Source: CAD feature listing. Evaluate the final solid. Frame: model axes, mm. Face numbers are marked on the shaded views. A direction names the side the tool comes from. Coordinates: 2 decimals unless noted, no trailing zeros. Loops run counter-clockwise (first coordinate to the right, second up) from the corner with the lowest first, then second, coordinate; pieces in that order, holes last.
Item 1: Reachability of the marked faces 1, 2 and 3 from +Z, -Z, +X, -X, +Y, -Y: full face, straight path, thin tool, end or side. Return the list, or none.
Item 2: Pin query (flat end, axial travel): pin 1 Ø8 at (x, y) = (9.5, -2.5) entering from +Z. Return the tip coordinate at first contact, or that it passes through.
Item 3: Line query: probe 1 along X at (y, z) = (-3.25, 11.25) (3 decimals); probe 2 along Y at (x, z) = (3.5, 7.5); probe 3 along Y at (x, z) = (5.5, 9.25). Output: solid intervals per line, ascending.
Item 4: Section query D-D, the plane x = 0. Return the cut outline in (y, z), then the cut area to 3 significant figures.
Item 5: Pull-direction query (Z, two-part tool) for the marked faces 4, 5 and 6; classes: +Z half, -Z half, draft (parallel to the pull), parting line (faces both ways), or undercut.
Item 6: Section query B-B, the plane x = -6.5. Return the cut outline in (y, z), then the cut area to 3 significant figures.
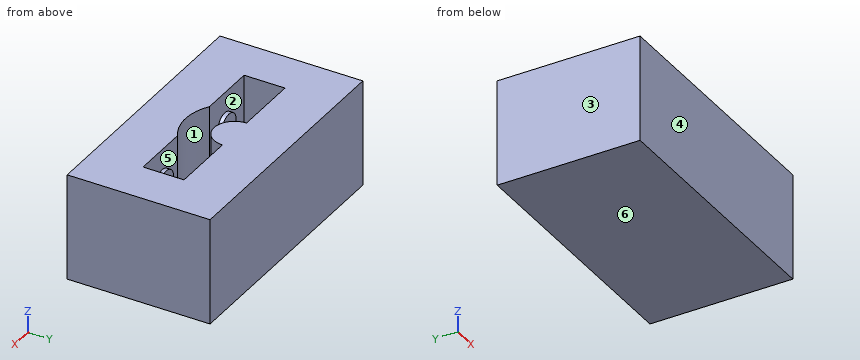
```python
from build123d import *

# Parameters (mm, degrees)
SKETCH1_R      = 24
EXTRUDE1_DEPTH = 5
SKETCH2_R      = 24
EXTRUDE2_DEPTH = 8
SKETCH9_R      = 24
SKETCH9_W      = 31.75
SKETCH9_H      = 17.4625
EXTRUDE4_DEPTH = 13
SKETCH11_R     = 1.5
EXTRUDE6_DEPTH = 0.5


with BuildPart() as part:
    # Sketch1 → Extrude1 (new body)
    with BuildSketch(Plane.XY):
        Circle(SKETCH1_R)
    extrude(amount=EXTRUDE1_DEPTH)

    # Sketch2 → Extrude2 (add)
    with BuildSketch(Plane.XY.offset(5)):
        Circle(SKETCH2_R)
        with BuildLine():
            Line((-2.5, 0), (-10.5, 0))
            Line((-10.5, 0), (-10.5, -5))
            Line((-10.5, -5), (-3.31662479, -5))
            ThreePointArc((-3.31662479, -5), (0, -6), (3.31662479, -5))
            Line((3.31662479, -5), (10.5, -5))
            Line((10.5, -5), (10.5, 0))
            Line((10.5, 0), (2.5, 0))
            ThreePointArc((2.5, 0), (0, -2.5), (-2.5, 0))
        make_face(mode=Mode.SUBTRACT)
    extrude(amount=EXTRUDE2_DEPTH)

    # Sketch9 → Extrude4 (cut)
    with BuildSketch(Plane.XY.offset(13)):
        Circle(SKETCH9_R)
        with Locations((0, -2.38125)):
            Rectangle(SKETCH9_W, SKETCH9_H, mode=Mode.SUBTRACT)
    extrude(amount=-EXTRUDE4_DEPTH, mode=Mode.SUBTRACT)

    # Sketch11 → Extrude6 (add)
    with BuildSketch(Plane(origin=(0, -5, 0), x_dir=(1, 0, 0), z_dir=(0, 1, 0))):
        with Locations((-6.5, -9)):
            Circle(SKETCH11_R)
        with Locations((6.5, -9)):
            Circle(SKETCH11_R)
    extrude(amount=EXTRUDE6_DEPTH)


solid = part.part
```
Verdict:
1. face 1: +Z
1. face 2: none
1. face 3: +Z, -Z, -X, +Y, -Y
2. pin 1: stops at z = 13
3. probe 1: x = -15.875 to -10.5, 10.5 to 15.875
3. probe 2: y = -11.11 to -5, 0 to 6.35
3. probe 3: y = -11.11 to -4.5, 0 to 6.35
4. outline: (-11.11, 0) - (6.35, 0) - (6.35, 13) - (-2.5, 13) - (-2.5, 5) - (-6, 5) - (-6, 13) - (-11.11, 13) - close
4. area: 199 mm2
5. face 4: draft
5. face 5: undercut
5. face 6: -Z half
6. outline: (-11.11, 0) - (6.35, 0) - (6.35, 13) - (0, 13) - (0, 5) - (-5, 5) - (-5, 7.5) - (-4.5, 7.5) - (-4.5, 10.5) - (-5, 10.5) - (-5, 13) - (-11.11, 13) - close
6. area: 189 mm2
